Read the model definition and answer for the solid it produces. Units are mm, in the model's axes. Coordinates: 2 decimals unless noted, no trailing zeros. Answer in a Markdown table with one row per item.
from build123d import *

# Parameters (mm, degrees)
SKETCH1_R           = 6.35
BOSS_EXTRUDE1_DEPTH = 1.5875
SKETCH2_R           = 1.5875
CUT_EXTRUDE1_DEPTH  = 76.374385622
FILLET1_R           = 0.2


with BuildPart() as part:
    # Sketch1 → Boss-Extrude1 (new body)
    with BuildSketch(Plane.XY):
        with Locations((68.398246491, 3.214386977)):
            Circle(SKETCH1_R)
    extrude(amount=BOSS_EXTRUDE1_DEPTH)

    # Sketch2 → Cut-Extrude1 (cut, through all)
    with BuildSketch(Plane(origin=(0, 0, 0), x_dir=(-1, 0, 0), z_dir=(0, 0, -1))):
        with Locations((-68.398246491, 3.214386977)):
            Circle(SKETCH2_R)
    extrude(amount=-CUT_EXTRUDE1_DEPTH, mode=Mode.SUBTRACT)

    # Fillet1
    fillet1_edges = [part.edges().sort_by_distance(p)[0] for p in [
        (62.048246491, 3.214386977, 0),
        (62.048246491, 3.214386977, 1.5875),
        (69.985746491, 3.214386977, 1.5875),
        (69.985746491, 3.214386977, 0),
    ]]
    fillet(fillet1_edges, radius=FILLET1_R)


solid = part.part
Q1. For a pull along X with two mould halves and no side action, classify faces 1 (the face through (69.568, 4.287, 0.785)), 2 (the face through (70, 2, 1.588)), 3 (the face through (74.264, 0.782, 0.785)) as pulls with the +X half, pulls with the -X half, needs draft (parallel to the pull), parting line crosses it, or undercut.
Outcome:
| item | result |
|---|---|
| face 1 | undercut |
| face 2 | needs draft |
| face 3 | parting line crosses it |
Q2. Consider line 1 (Y direction, x = 68.5, z = 1.35); line 2 (Y direction, x = 68, z = 0.9); line 3 (Y direction, x = 64.25, z = 0.5). Determine where each line is inside the solid, lowest interval first.
Outcome:
| item | result |
|---|---|
| line 1 | -3.13 to 1.63, 4.8 to 9.56 |
| line 2 | -3.12 to 1.68, 4.75 to 9.55 |
| line 3 | -1.59 to 8.02 |
Q3. Given pin 1 (2.5 mm diameter, centred on x = 68.4, y = 3.21, fed in from -Z), flat-ended and moving along its own axis, determine where the tip first touches the part or whether it passes through.
Outcome:
| item | result |
|---|---|
| pin 1 | through |
